CAD build for the part. Positions are in the model's coordinates, mm. A direction names the side the tool comes from. Round coordinates to 2 decimals unless told otherwise and drop trailing zeros. Write each loop counter-clockwise with the first axis right and the second up, starting at its lowest first coordinate (ties: lowest second). Pieces come first, ordered by that corner, then holes. Notation, with made-up numbers: M 29,0.5 L 82,0.5 A29 cw 82,28.5 Z; hole C 67,68.5 d2. An arc over 180 degrees is marked long. Write each question's results on one line, items separated by ' | '. Start each with the question number.
```python
from build123d import *

# Parameters (mm, degrees)
F1_DEPTH = 3.175
F3_D     = 3.4544
F3_DEPTH = 12.7
F3_TIP   = 1.0378064612
F5_D     = 3.175


with BuildPart() as f1:
    # F0 (on Top) → F1 (new body, symmetric)
    with BuildSketch(Plane.XY):
        with BuildLine():
            Line((0, -3.175), (-6.985, -3.175))
            Line((-6.985, -3.175), (-6.985, -6.35))
            Line((-6.985, -6.35), (5.715, -6.35))
            ThreePointArc((5.715, -6.35), (6.6449359697, -4.1049359697), (8.89, -3.175))
            Line((8.89, -3.175), (18.415, -3.175))
            Line((18.415, -3.175), (18.415, 3.175))
            Line((18.415, 3.175), (8.89, 3.175))
            ThreePointArc((8.89, 3.175), (6.6449359697, 4.1049359697), (5.715, 6.35))
            Line((5.715, 6.35), (-6.985, 6.35))
            Line((-6.985, 6.35), (-6.985, 3.175))
            Line((-6.985, 3.175), (0, 3.175))
            ThreePointArc((0, 3.175), (3.175, 0), (0, -3.175))
        make_face()
    extrude(amount=F1_DEPTH, both=True)

    # F3
    with Locations(Plane.YZ.offset(18.415)):
        with Locations((0, 0)):
            Hole(F3_D / 2, depth=F3_DEPTH)
            with Locations((0, 0, -(F3_DEPTH + F3_TIP / 2))):  # 118° drill point
                Cone(0, F3_D / 2, F3_TIP, mode=Mode.SUBTRACT)

    # F5 (through all)
    with Locations(Plane.XZ.offset(6.35)):
        with Locations((-3.81, 0)):
            Hole(F5_D / 2)


solid = f1.part
```
1) Saw through at C-C, the plane x = 12.75. Write the cut outline in (y, z) (3 decimals), plus the area to 3 significant figures.
2) Saw through at D-D, the plane x = 0.5. Write the cut outline in (y, z) (3 decimals), plus the area to 3 significant figures.
3) 3-axis set-ups, long thin cutter, end or side, ignore diameter. For faces 1 (the face through (14, 3.175, 0)), 2 (the face through (6, 0, 3.175)), 3 (the face through (11.976, 0.225, 1.713)), 4 (the face through (-2, -3.175, 0)): which of +Z, -Z, +X, -X, +Y, -Y reach the whole face in a straight line?
4) Saw through at B-B, the plane z = 2.25. Write the cut outline in (x, y) (3 decimals).
5) Wall check: line 1 along Y through (x, z) = (-2.75, -2) (3 decimals); line 2 along Y through (x, z) = (10.5, 0) (3 decimals). Give the ranges that are in metal, low to high. Write a range as from..to.
6) Drop flat-ended pins along their axis: pin 1 Ø3 at (y, z) = (0, 0) entering from +X; pin 2 Ø2 at (x, z) = (12, -1.5) entering from -Y (3 decimals); pin 3 Ø3 at (x, z) = (-3.81, 0) entering from -Y. Give the stop position or say it passes through.
7) Pull direction X, two halves, no side cores. Call faces 5 (the face through (14, -3.175, 0)), 6 (the face through (-6.985, -5, 0)), 7 (the face through (-5.276, 4.785, -0.608)), 8 (the face through (-5.276, -4.74, -0.608)): pulls with the +X half, pulls with the -X half, needs draft (parallel to the pull), parting line crosses it, or undercut.
8) Saw through at A-A, the plane x = -3.81. State how many separate pieces and enclosed holes the cut face has, plus the area to 3 significant figures.
Filled sheet:
1) outline: M -3.175,-3.175 L 3.175,-3.175 L 3.175,3.175 L -3.175,3.175 Z; hole C 0,0 d3.454 | area: 31.0 mm^2
2) outline: M -6.35,-3.175 L -3.135,-3.175 L -3.135,3.175 L -6.35,3.175 Z; M 3.135,-3.175 L 6.35,-3.175 L 6.35,3.175 L 3.135,3.175 Z | area: 40.8 mm^2
3) face 1: +Z, -Z, +X, +Y | face 2: +Z, +X, -X, +Y, -Y | face 3: +X | face 4: +Z, -Z, -X
4) outline: M -6.985,-6.35 L 5.715,-6.35 A3.175 cw 8.89,-3.175 L 18.415,-3.175 L 18.415,3.175 L 8.89,3.175 A3.175 cw 5.715,6.35 L -6.985,6.35 L -6.985,3.175 L 0,3.175 A3.175 cw 0,-3.175 L -6.985,-3.175 Z
5) line 1: y = -6.35..-3.175, 3.175..6.35 | line 2: y = -3.175..-1.727, 1.727..3.175
6) pin 1: stops at x = 5.58 | pin 2: stops at y = -3.175 | pin 3: passes through
7) face 5: needs draft | face 6: pulls with the -X half | face 7: undercut | face 8: undercut
8) separate pieces: 4 | enclosed holes: 0 | area: 20.2 mm^2
